Can you work these out from the model? Positions are in its coordinate system, mm. Face numbers are marked on the shaded views. A direction names the side the tool comes from. Round coordinates to 2 decimals unless told otherwise and drop trailing zeros. Loops run counter-clockwise (first coordinate to the right, second up) from the corner with the lowest first, then second, coordinate; pieces in that order, holes last. Notation, with made-up numbers: M 79.5,43 L 117.5,43 A6 ccw 117.5,48 Z; hole C -13.5,-22.75 d9. An arc over 180 degrees is marked long. Answer as CSV lines item,"result".
from build123d import *

# Parameters (mm, degrees)
S_BOX1_W       = 8
S_BOX1_H       = 2.5
BOSS_1_DEPTH   = 20
S_BOX2_W       = 7
S_BOX2_H       = 36.2
BOSS_2_DEPTH   = 28
S_HOLE3_R      = 1.25
HOLE_3_DEPTH   = 2.7
S_CUT4_W       = 7.2
S_CUT4_H       = 3
POCKET_4_DEPTH = 14.1
S_CUT5_W       = 7.2
S_CUT5_H       = 3
POCKET_5_DEPTH = 14.1


with BuildPart() as part:
    # S_box1 → Boss_1 (new body)
    with BuildSketch(Plane.XY.offset(-16)):
        with Locations((0, 3.25)):
            Rectangle(S_BOX1_W, S_BOX1_H)
    extrude(amount=BOSS_1_DEPTH)

    # S_box2 → Boss_2 (add)
    with BuildSketch(Plane.XY.offset(-44)):
        with Locations((-0.5, -13.6)):
            Rectangle(S_BOX2_W, S_BOX2_H)
    extrude(amount=BOSS_2_DEPTH)

    # S_hole3 → Hole_3 (cut)
    with BuildSketch(Plane(origin=(0, 1.9, 0), x_dir=(1, 0, 0), z_dir=(0, 1, 0))):
        with Locations(Location((0, 0, 0), (0, 0, 90))):
            Circle(S_HOLE3_R)
    extrude(amount=HOLE_3_DEPTH, mode=Mode.SUBTRACT)

    # S_cut4 → Pocket_4 (cut)
    with BuildSketch(Plane.XY.offset(-44.1)):
        with Locations((-0.5, -7.07)):
            Rectangle(S_CUT4_W, S_CUT4_H)
    extrude(amount=POCKET_4_DEPTH, mode=Mode.SUBTRACT)

    # S_cut5 → Pocket_5 (cut)
    with BuildSketch(Plane.XY.offset(-44.1)):
        with Locations((-0.5, -20.13)):
            Rectangle(S_CUT5_W, S_CUT5_H)
    extrude(amount=POCKET_5_DEPTH, mode=Mode.SUBTRACT)


solid = part.part
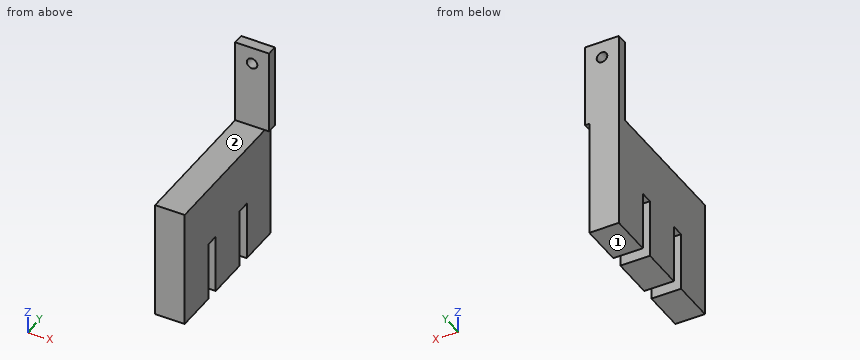
Item 1: Will these pins go through, and if not, where does the flat tip stop? pin 1 (2 mm diameter, centred on x = 1, y = -15, fed in from +Z); pin 2 (1.5 mm diameter, centred on y = -2, z = -19, fed in from +X); pin 3 (0.5 mm diameter, centred on x = 3.5, y = 3, fed in from -Z).
Output:
pin 1,"stops at z = -16"
pin 2,"stops at x = 3"
pin 3,"stops at z = -16"
Item 2: If we section it at C-C on z = 0: Write out the boundary of the cut face in (x, y), then the cut area to 4 significant figures.
Output:
outline,"M -4,2 L -1.25,2 L -1.25,4.5 L -4,4.5 Z; M 1.25,2 L 4,2 L 4,4.5 L 1.25,4.5 Z"
area,"13.75 mm2"
Item 3: If we section it at D-D on x = -2.5: Write out the boundary of the cut face in (y, z), then the cut area to 3 significant figures.
Output:
outline,"M -31.7,-44 L -21.63,-44 L -21.63,-30 L -18.63,-30 L -18.63,-44 L -8.57,-44 L -8.57,-30 L -5.57,-30 L -5.57,-44 L 4.5,-44 L 4.5,4 L 2,4 L 2,-16 L -31.7,-16 Z"
area,"980 mm2"
Item 4: If we section it at B-B on z = -40: Write out the boundary of the cut face in (x, y), then the cut area to 3 significant figures.
Output:
outline,"M -4,-31.7 L 3,-31.7 L 3,-21.63 L -4,-21.63 Z; M -4,-18.63 L 3,-18.63 L 3,-8.57 L -4,-8.57 Z; M -4,-5.57 L 3,-5.57 L 3,4.5 L -4,4.5 Z"
area,"211 mm2"
Item 5: If we section it at A-A on x = 0: Write out the boundary of the cut face in (y, z).
Output:
outline,"M -31.7,-44 L -21.63,-44 L -21.63,-30 L -18.63,-30 L -18.63,-44 L -8.57,-44 L -8.57,-30 L -5.57,-30 L -5.57,-44 L 4.5,-44 L 4.5,-1.25 L 2,-1.25 L 2,-16 L -31.7,-16 Z; M 2,1.25 L 4.5,1.25 L 4.5,4 L 2,4 Z"
Item 6: On a 3-axis mill with a long thin cutter (end or side, diameter ignored), from which of +Z, -Z, +X, -X, +Y, -Y can I reach the whole of each face in a straight line? I mean the marked faces 1 and 2. Say none if no direction works.
Output:
face 1,"-Z, +X, -X, +Y, -Y"
face 2,"+Z, +X, -X, -Y"
Item 7: If I drill on line 1 along Y through (x, z) = (1, -33.5); line 2 along X through (y, z) = (3.2, 0); line 3 along Y through (x, z) = (-2, 2), over which ranges is the centre line in solid material (lowest first)? Write a range as from..to.
Output:
line 1,"y = -31.7..-21.63, -18.63..-8.57, -5.57..4.5"
line 2,"x = -4..-1.25, 1.25..4"
line 3,"y = 2..4.5"
